```python
from build123d import *

# Parameters (mm, degrees)
F0_R     = 26.5
F0_R_2   = 6.5
F1_DEPTH = 9
F2_R     = 8
F3_SIZE  = 8


with BuildPart() as f1:
    # F0 (on Top) → F1 (new body)
    with BuildSketch(Plane.XY):
        Circle(F0_R)
        Circle(F0_R_2, mode=Mode.SUBTRACT)
    extrude(amount=F1_DEPTH)

    # F2
    f2_edges = [f1.edges().sort_by_distance(p)[0] for p in [
        (-26.5, 0, 9),
    ]]
    fillet(f2_edges, radius=F2_R)

    # F3
    f3_edges = [f1.edges().sort_by_distance(p)[0] for p in [
        (-6.5, 0, 9),
    ]]
    chamfer(f3_edges, length=F3_SIZE)


solid = f1.part
```
For this review, take the finished solid that the model builds, in its own axes (mm). Give positions to 0.01 mm unless a question says otherwise; leave off trailing zeros. Loops run counter-clockwise (first coordinate to the right, second up) from the corner with the lowest first, then second, coordinate; pieces in that order, holes last. Notation, with made-up numbers: M -23.5,53 L 16.5,53 A16 ccw 16.5,82 Z; hole C 89.5,37 d11. An arc over 180 degrees is marked long. One line per item, written item: value. Start each with the question number.
Q1. Add section C-C (z = 7.75). Give the boundary of the cut face in (x, y), and give its area (3 significant figures).
Q2. Clearance check with flat-ended pins moving along their axes: pin 1 Ø2 at (x, z) = (11, 6) entering from +Y; pin 2 Ø4 at (x, z) = (5.5, 5) entering from +Y; pin 3 Ø2 at (x, z) = (-12, 3) entering from -Y. State where each tip first meets the part, or that it passes through.
Q3. For L1, parallel to Y at x = 0, z = 0.7; L2, parallel to X at y = 10.5, z = 7.75; L3, parallel to Y at x = 1, z = 3.25, list the stretches that pass through material, from the lowest coordinate up.
Q4. Add section A-A (x = 0). Give the boundary of the cut face in (y, z), and give its area (3 significant figures).
Q5. Draft analysis for pull direction X (two halves, no side actions). For faces 1 (the face through (14.246, 22.345, 0.493)), 2 (the face through (-5.158, -3.955, 0.493)), 3 (the face through (-11, -10, 9)), state which applies: released by +X, released by -X, zero draft, split by the parting line, or undercut.
Q6. Add section D-D (z = 1.75). Give the boundary of the cut face in (x, y).
Reply:
1. outline: C 0,0 d45.59; hole C 0,0 d26.5
1. area: 1,080 mm²
2. pin 1: y = 23.07
2. pin 2: y = 25.78
2. pin 3: y = -23.89
3. L1: -26.5 to -6.5, 6.5 to 26.5
3. L2: -20.23 to -8.08, 8.08 to 20.23
3. L3: -26.16 to -8.69, 8.69 to 26.16
4. outline: M -26.5,0 L -6.5,0 L -6.5,1 L -14.5,9 L -18.5,9 A8 ccw -26.5,1 Z; M 6.5,0 L 26.5,0 L 26.5,1 A8 ccw 18.5,9 L 14.5,9 L 6.5,1 Z
4. area: 269 mm²
5. face 1: split by the parting line
5. face 2: undercut
5. face 3: zero draft
6. outline: C 0,0 d52.93; hole C 0,0 d14.5
